```python
from build123d import *

# Parameters (mm, degrees)
BOSS_EXTRUDE1_DEPTH      = 4.7625
BOSS_EXTRUDE1_DEPTH_BACK = 4.7625
CHAMFER1_SIZE            = 0.13890625
FILLET1_R                = 0.13890625


with BuildPart() as part:
    # Sketch3 → Revolve1 (revolve)
    with BuildSketch(Plane(origin=(0, 0, 0), x_dir=(0, 0, -1), z_dir=(1, 0, 0)), mode=Mode.PRIVATE) as revolve1_sk:
        Polygon((11.1125, 0), (-11.1125, 0), (-11.1125, 0.94615), (-10.63625, 1.4224), (-5.9944, 1.4224), (-5.5245, 0.9525), (-4.7625, 0.9525), (-4.7625, 2.778125), (4.7625, 2.778125), (4.7625, 0.9525), (5.5245, 0.9525), (5.9944, 1.4224), (10.63625, 1.4224), (11.1125, 0.94615), align=None)
    revolve(revolve1_sk.sketch.rotate(Axis((0, 0, 11.1125), (0, 0, -1)), 90), axis=Axis((0, 0, 11.1125), (0, 0, -1)))

    # Sketch4 → Boss-Extrude1 (add, two sides: drawn at the far end of the back side and taken through both)
    with BuildSketch(Plane.XY.offset(-BOSS_EXTRUDE1_DEPTH_BACK)):
        Polygon((-3.207902433, 0), (-1.603951217, -2.778125), (1.603951217, -2.778125), (3.207902433, 0), (1.603951217, 2.778125), (-1.603951217, 2.778125), align=None)
    extrude(amount=BOSS_EXTRUDE1_DEPTH + BOSS_EXTRUDE1_DEPTH_BACK)

    # Chamfer1
    chamfer1_edges = [part.edges().sort_by_distance(p)[0] for p in [
        (2.405926825, 1.3890625, 4.7625),
        (0, 2.778125, 4.7625),
        (-2.405926825, 1.3890625, 4.7625),
        (-2.405926825, -1.3890625, 4.7625),
        (0, -2.778125, 4.7625),
        (2.405926825, -1.3890625, 4.7625),
        (-2.405926825, 1.3890625, -4.7625),
        (0, 2.778125, -4.7625),
        (2.405926825, 1.3890625, -4.7625),
        (2.405926825, -1.3890625, -4.7625),
        (0, -2.778125, -4.7625),
        (-2.405926825, -1.3890625, -4.7625),
    ]]
    chamfer(chamfer1_edges, length=CHAMFER1_SIZE)

    # Fillet1
    fillet1_edges = [part.edges().sort_by_distance(p)[0] for p in [
        (-0.9525, 0, -4.7625),
        (-0.9525, 0, 4.7625),
        (-3.207902433, 0, 0),
        (-1.603951217, 2.778125, 0),
        (-1.603951217, -2.778125, 0),
        (1.603951217, -2.778125, 0),
        (3.207902433, 0, 0),
        (1.603951217, 2.778125, 0),
    ]]
    fillet(fillet1_edges, radius=FILLET1_R)


solid = part.part
```
Geometry check sheet. Reference: the model listing, model coordinates, mm. A direction names the side the tool comes from. Give positions to 0.01 mm unless a question says otherwise; leave off trailing zeros. Write each loop counter-clockwise with the first axis right and the second up, starting at its lowest first coordinate (ties: lowest second). Pieces come first, ordered by that corner, then holes. Notation, with made-up numbers: (35.5, -28.5) -> (65.5, -28.5) arc R17 ccw to (65.5, -22.5) -> close; hole circle Ø3 at (47, -7). An arc over 180 degrees is marked (long way). Use one line per item in the form item = value.
Item 1: Depth check by flat-ended pin: pin 1 Ø2 at (x, y) = (-0.5, -1) entering from -Z. Enter the tip coordinate at first touch or a pass-through.
Results list:
pin_1 = -11.11
Item 2: Sectioned sample at C-C on y = 1.65. Enter the section's corners in (x, z).
Results list:
outline = (-2.26, -4.62) -> (-2.09, -4.76) -> (2.09, -4.76) -> (2.26, -4.62) -> (2.26, 4.62) -> (2.09, 4.76) -> (-2.09, 4.76) -> (-2.26, 4.62) -> close
Item 3: Access from +Z, -Z, +X, -X, +Y, -Y to the whole of each face (thin tool, end or side, straight path). Record for faces 1 (the flat face through (0, -2.778, 0)), 2 (the cylindrical face through (-0.124, -0.944, -5.217)), 3 (the cylindrical face through (0.66, 1.26, 8.28)).
Results list:
face_1 = +Z, -Z, +X, -X, -Y
face_2 = none
face_3 = +Z
Item 4: Scan lines: line 1 (Z direction, x = 1, y = 0.85); line 2 (Z direction, x = -1, y = 1.9); line 3 (X direction, y = 0.1, z = 8.5). Record each from-to range of solid material in increasing order.
Results list:
line_1 = -10.75 to -5.88, -4.76 to 4.76, 5.88 to 10.75
line_2 = -4.76 to 4.76
line_3 = -1.42 to 1.42
Item 5: Sectioned sample at A-A on z = 2.75. Enter the section's corners in (x, y).
Results list:
outline = (-3.17, -0.07) -> (-1.64, -2.71) arc R0.14 ccw to (-1.52, -2.78) -> (1.52, -2.78) arc R0.14 ccw to (1.64, -2.71) -> (3.17, -0.07) arc R0.14 ccw to (3.17, 0.07) -> (1.64, 2.71) arc R0.14 ccw to (1.52, 2.78) -> (-1.52, 2.78) arc R0.14 ccw to (-1.64, 2.71) -> (-3.17, 0.07) arc R0.14 ccw to start
